Geometry check sheet. Reference: the model listing, model coordinates, mm. Round coordinates to 2 decimals unless told otherwise and drop trailing zeros. Loops run counter-clockwise (first coordinate to the right, second up) from the corner with the lowest first, then second, coordinate; pieces in that order, holes last. Notation, with made-up numbers: (29.5, 44) - (79.5, 44) arc R25 cw to (79.5, 79) - close; hole circle Ø5 at (-18.5, 13.25). An arc over 180 degrees is marked (long way). Answer as CSV lines item,"result". Start each with the question number.
1) Cross-section at D-D on z = 75.5. Record the boundary of the cut face in (x, y), and give its area (3 significant figures).
2) Thickness scan on line 1 along Y through (x, z) = (-66, 117); line 2 along Z through (x, y) = (-69.5, -1.5); line 3 along Y through (x, z) = (-63.5, 75.5). Record the ranges inside material, lowest first.
3) Cross-section at B-B on z = 12.5. Record the boundary of the cut face in (x, y).
4) Cross-section at C-C on y = -9.25. Record the boundary of the cut face in (x, z), and give its area (3 significant figures).
5) Depth check by flat-ended pin: P1, Ø6, axis at y = -9, z = 98, coming from the -X side; P2, Ø5, axis at x = -69, z = 53.5, coming from the +Y side; P3, Ø3, axis at x = -64, z = 75.5, coming from the +Y side. Enter the tip coordinate at first touch or a pass-through.
6) Cross-section at A-A on x = -70. Record the boundary of the cut face in (y, z), and give its area (3 significant figures).
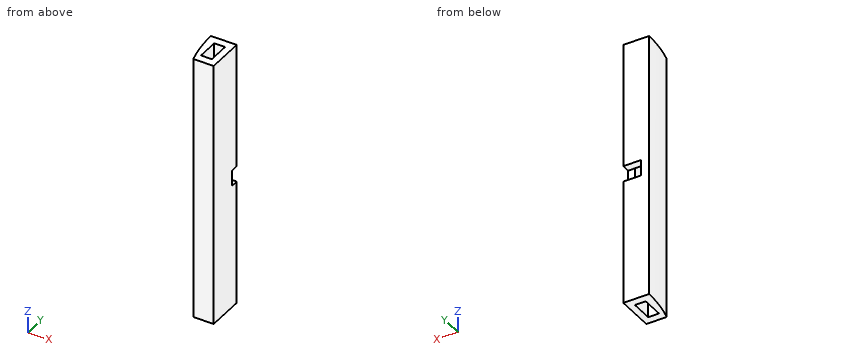
from build123d import *

# Parameters (mm, degrees)
BOSS_EXTRUDE1_DEPTH = 149.86
SKETCH2_W           = 9.906
SKETCH2_H           = 4.4958
BOSS_EXTRUDE2_DEPTH = 70.4596
SKETCH3_W           = 9.906
SKETCH3_H           = 4.4958
BOSS_EXTRUDE3_DEPTH = 70.4596


with BuildPart() as part:
    # Sketch1 → Boss-Extrude1 (new body)
    with BuildSketch(Plane.XY):
        with BuildLine():
            Line((-61.5779714, -4.4958), (-65.3879714, -4.4958))
            Line((-65.3879714, -4.4958), (-65.3879714, -16.6878))
            Line((-65.3879714, -16.6878), (-71.4839714, -16.6878))
            Line((-71.4839714, -16.6878), (-71.4839714, 0))
            Line((-71.4839714, 0), (-76.073, 0))
            ThreePointArc((-76.073, 0), (-75.317007822, -10.698114871), (-73.064056964, -21.1836))
            Line((-73.064056964, -21.1836), (-61.5779714, -21.1836))
            Line((-61.5779714, -21.1836), (-61.5779714, -4.4958))
        make_face()
    extrude(amount=BOSS_EXTRUDE1_DEPTH)

    # Sketch2 → Boss-Extrude2 (add)
    with BuildSketch(Plane.XY.offset(149.86)):
        with Locations((-66.5309714, -2.2479)):
            Rectangle(SKETCH2_W, SKETCH2_H)
    extrude(amount=-BOSS_EXTRUDE2_DEPTH)

    # Sketch3 → Boss-Extrude3 (add)
    with BuildSketch(Plane(origin=(0, 0, 0), x_dir=(-1, 0, 0), z_dir=(0, 0, -1))):
        with Locations((66.5309714, -2.2479)):
            Rectangle(SKETCH3_W, SKETCH3_H)
    extrude(amount=-BOSS_EXTRUDE3_DEPTH)


solid = part.part
Answer block:
1,outline,"(-76.07, 0) arc R76.07 ccw to (-73.06, -21.18) - (-61.58, -21.18) - (-61.58, -4.5) - (-65.39, -4.5) - (-65.39, -16.69) - (-71.48, -16.69) - (-71.48, 0) - close"
1,area,"167 mm^2"
2,line 1,"y = -21.18 to -16.69, -4.5 to 0"
2,line 2,"z = 0 to 70.46, 79.4 to 149.86"
2,line 3,"y = -21.18 to -4.5"
3,outline,"(-76.07, 0) arc R76.07 ccw to (-73.06, -21.18) - (-61.58, -21.18) - (-61.58, 0) - close; hole (-71.48, -16.69) - (-65.39, -16.69) - (-65.39, -4.5) - (-71.48, -4.5) - close"
4,outline,"(-75.51, 0) - (-71.48, 0) - (-71.48, 149.86) - (-75.51, 149.86) - close; (-65.39, 0) - (-61.58, 0) - (-61.58, 149.86) - (-65.39, 149.86) - close"
4,area,"1,170 mm^2"
5,P1,"stops at x = -75.84"
5,P2,"stops at y = 0"
5,P3,"stops at y = -4.5"
6,outline,"(-21.18, 0) - (-16.69, 0) - (-16.69, 149.86) - (-21.18, 149.86) - close; (-4.5, 0) - (0, 0) - (0, 70.46) - (-4.5, 70.46) - close; (-4.5, 79.4) - (0, 79.4) - (0, 149.86) - (-4.5, 149.86) - close"
6,area,"1,310 mm^2"
